```python
from build123d import *

# Parameters (mm, degrees)
SKETCH_R      = 2.05
EXTRUDE_DEPTH = 5
CHAMFER_SIZE  = 2


with BuildPart() as part:
    # Sketch → Extrude (new body)
    with BuildSketch(Plane.XY):
        Polygon((0, 0), (0, 40), (20, 40), (20, 20), (40, 20), (40, 0), align=None)
        with Locations((10, 10)):
            Circle(SKETCH_R, mode=Mode.SUBTRACT)
        with Locations((30, 10)):
            Circle(SKETCH_R, mode=Mode.SUBTRACT)
        with Locations((10, 30)):
            Circle(SKETCH_R, mode=Mode.SUBTRACT)
    extrude(amount=EXTRUDE_DEPTH)

    # Chamfer
    chamfer_edges = [part.edges().sort_by_distance(p)[0] for p in [
        (0, 20, 5),
        (10, 40, 5),
        (20, 30, 5),
        (30, 20, 5),
        (40, 10, 5),
        (20, 0, 5),
    ]]
    chamfer(chamfer_edges, length=CHAMFER_SIZE)


solid = part.part
```
For this review, take the finished solid that the model builds, in its own axes (mm). A direction names the side the tool comes from. Round coordinates to 2 decimals unless told otherwise and drop trailing zeros. Order: outer loops, then holes, each group sorted by start corner. A loop starts at its lowest first (then second) coordinate and runs counter-clockwise, first axis right, second up. Notation, with made-up numbers: (-7, 77) -> (50, 77) arc R16 ccw to (50, 89) -> close; hole circle Ø11 at (39, 23.5). An arc over 180 degrees is marked (long way). Use a Markdown table: item, result.
Item 1: Take a section at C-C (z = 3.9). State the section outline as (x, y) points, plus the area to 3 significant figures.
Resolved:
| item | result |
|---|---|
| outline | (0.9, 0.9) -> (39.1, 0.9) -> (39.1, 19.1) -> (19.1, 19.1) -> (19.1, 39.1) -> (0.9, 39.1) -> close; hole circle Ø4.1 at (10, 10); hole circle Ø4.1 at (10, 30); hole circle Ø4.1 at (30, 10) |
| area | 1,020 mm² |
Item 2: Take a section at D-D (y = 10). State the section outline as (x, z) points.
Resolved:
| item | result |
|---|---|
| outline | (0, 0) -> (7.95, 0) -> (7.95, 5) -> (2, 5) -> (0, 3) -> close; (12.05, 0) -> (27.95, 0) -> (27.95, 5) -> (12.05, 5) -> close; (32.05, 0) -> (40, 0) -> (40, 3) -> (38, 5) -> (32.05, 5) -> close |
Item 3: Take a section at A-A (x = 30). State the section outline as (y, z) points.
Resolved:
| item | result |
|---|---|
| outline | (0, 0) -> (7.95, 0) -> (7.95, 5) -> (2, 5) -> (0, 3) -> close; (12.05, 0) -> (20, 0) -> (20, 3) -> (18, 5) -> (12.05, 5) -> close |
Item 4: For line 1 along Y through (x, z) = (10, 1.95); line 2 along Y through (x, z) = (30, 2.25); line 3 along Y through (x, z) = (8.5, 1.7), list the stretches that pass through material, from the lowest coordinate up. Write a range as [from, to].
Resolved:
| item | result |
|---|---|
| line 1 | y = [0, 7.95], [12.05, 27.95], [32.05, 40] |
| line 2 | y = [0, 7.95], [12.05, 20] |
| line 3 | y = [0, 8.6], [11.4, 28.6], [31.4, 40] |
Item 5: Draft analysis for pull direction X (two halves, no side actions). For faces 1 (the flat face through (16, 16, 5)), 2 (the cylindrical face through (28.373, 8.753, 2.465)), 3 (the flat face through (19, 29, 4)), state which applies: +X half, -X half, draft (parallel to the pull), parting line (faces both ways), or undercut.
Resolved:
| item | result |
|---|---|
| face 1 | draft |
| face 2 | undercut |
| face 3 | +X half |
Item 6: For pin 1 (1.5 mm diameter, centred on x = 34.5, z = 1, fed in from +Y), flat-tipped, find the tip position at first contact; note if it passes through.
Resolved:
| item | result |
|---|---|
| pin 1 | stops at y = 20 |
Item 7: Machinability: for faces 4 (the flat face through (29, 19, 4)), 5 (the cylindrical face through (8.373, 8.753, 2.465)), 6 (the flat face through (30, 20, 1)), which of the approach directions +Z, -Z, +X, -X, +Y, -Y give a long, thin tool a straight path to every point of the face, cutting with its end or side? Answer none if there is none.
Resolved:
| item | result |
|---|---|
| face 4 | +Z, +X, +Y |
| face 5 | +Z, -Z |
| face 6 | +Z, -Z, +X, +Y |
